Geometry check sheet. Reference: drawing and pictorial views, mm from the part's lowest x, y, z. A direction names the side the tool comes from. Round coordinates to 2 decimals unless told otherwise and drop trailing zeros. Write each loop counter-clockwise with the first axis right and the second up, starting at its lowest first coordinate (ties: lowest second). Pieces come first, ordered by that corner, then holes. Notation, with made-up numbers: (64.25, 59.5) - (101.25, 59.5) arc R21 cw to (101.25, 74.5) - close; hole circle Ø8 at (14.5, 70.25). An arc over 180 degrees is marked (long way). Return JSON: item names as keys, results as strings.
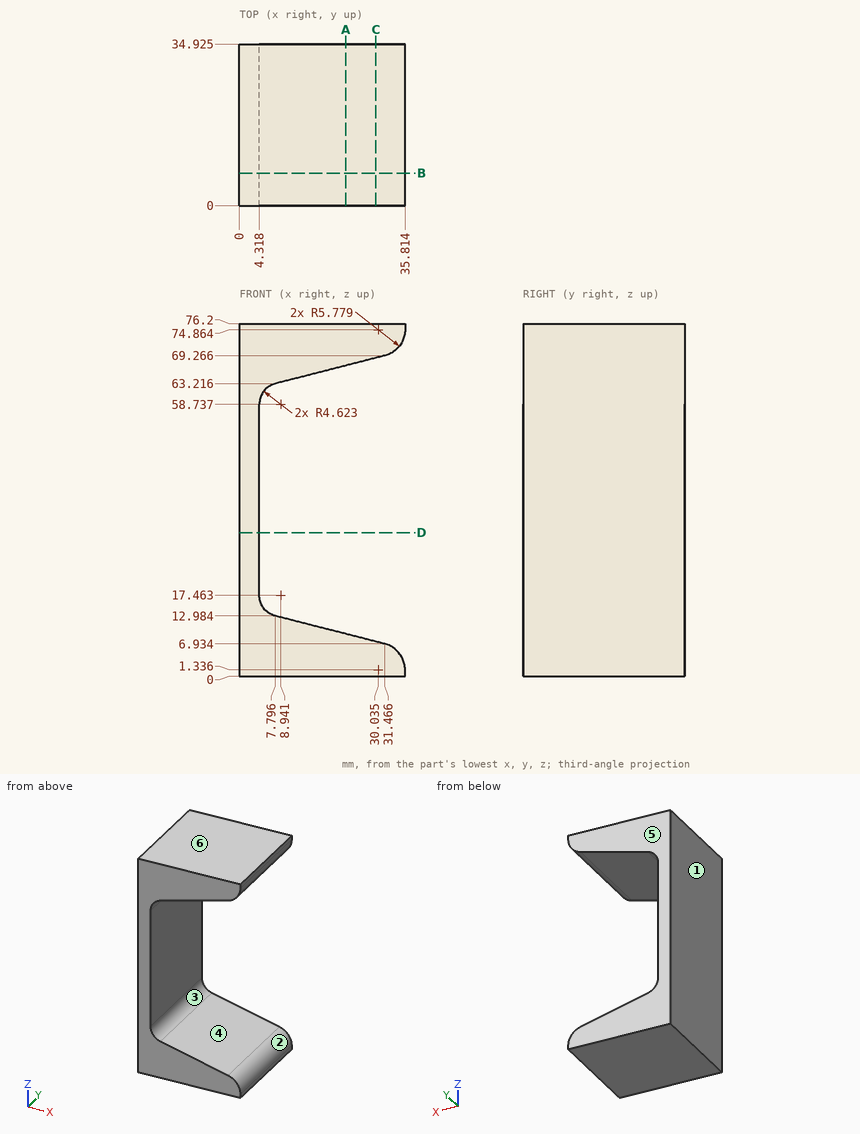
(1) Gauge pin test, flat end, axial feed: pin 1 (4 mm diameter, centred on y = 31.5, z = 57.5, fed in from +X). Record the tip position at first contact, or that the pin passes through.
Response values:
{"pin 1": "stops at x = 4.38"}
(2) Section check B-B, the plane y = 7. Enter the section's corners in (x, z) (1 decimal).
Response values:
{"outline": "(0, 0) - (35.8, 0) - (35.8, 1.3) arc R5.8 ccw to (31.5, 6.9) - (7.8, 13) arc R4.6 cw to (4.3, 17.5) - (4.3, 58.7) arc R4.6 cw to (7.8, 63.2) - (31.5, 69.3) arc R5.8 ccw to (35.8, 74.9) - (35.8, 76.2) - (0, 76.2) - close"}
(3) Section check A-A, the plane x = 23. Enter the section's corners in (y, z) (1 decimal).
Response values:
{"outline": "(0, 0) - (34.9, 0) - (34.9, 9.1) - (0, 9.1) - close; (0, 67.1) - (34.9, 67.1) - (34.9, 76.2) - (0, 76.2) - close"}
(4) Release check for a two-part mould opening along Z. For the marked faces 3, 4, 5 and 6 record: pulls with the +Z half, pulls with the -Z half, needs draft (parallel to the pull), parting line crosses it, or undercut.
Response values:
{"face 3": "undercut", "face 4": "undercut", "face 5": "needs draft", "face 6": "pulls with the +Z half"}
(5) Material ranges on line 1 along X through (y, z) = (25, 54.5); line 2 along Z through (x, y) = (20, 17) (1 decimal); line 3 along Z through (x, y) = (29.5, 28), recorded low to high. Write a range as [from, to].
Response values:
{"line 1": "x = [0, 4.32]", "line 2": "z = [0, 9.9], [66.3, 76.2]", "line 3": "z = [0, 7.44], [68.76, 76.2]"}
(6) Section check D-D, the plane z = 31. Enter the section's corners in (x, y) (1 decimal).
Response values:
{"outline": "(0, 0) - (4.3, 0) - (4.3, 34.9) - (0, 34.9) - close"}
(7) Access from +Z, -Z, +X, -X, +Y, -Y to the whole of each face (thin tool, end or side, straight path). Record for the marked faces 1 and 2.
Response values:
{"face 1": "+Z, -Z, -X, +Y, -Y", "face 2": "+X, +Y, -Y"}
(8) Section check C-C, the plane x = 29.5. Enter the section's corners in (y, z) (1 decimal).
Response values:
{"outline": "(0, 0) - (34.9, 0) - (34.9, 7.4) - (0, 7.4) - close; (0, 68.8) - (34.9, 68.8) - (34.9, 76.2) - (0, 76.2) - close"}
